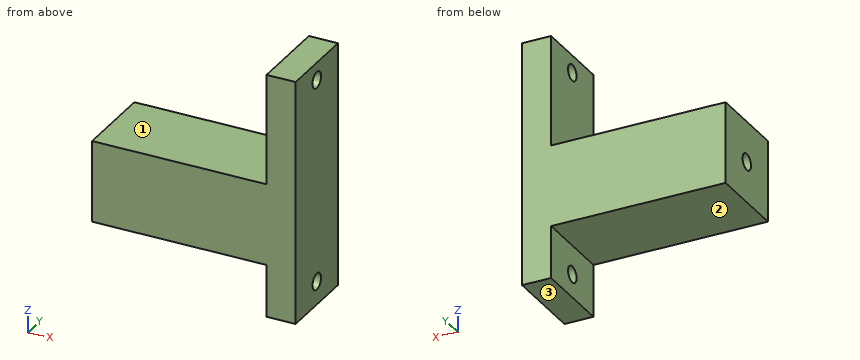
Autodesk Inventor part; units mm, degrees
ref_plane "YZ Plane" through (0, 0, 0) normal (1, 0, 0) x (0, 1, 0)
ref_plane "XZ Plane" through (0, 0, 0) normal (0, 1, 0) x (-1, 0, 0)
ref_plane "XY Plane" through (0, 0, 0) normal (0, 0, 1) x (1, 0, 0)
sketch "Sketch1" plane through (0, 0, 0) normal (1, 0, 0) x (0, 1, 0)
  line L0 (0, 0) -> (14, 0)
  line L1 (14, 0) -> (14, -42)
  line L2 (14, -42) -> (0, -42)
  line L3 (0, -42) -> (0, 0)
  line L4 (14, -19) -> (0, -19)
  line L5 (0, -19) -> (0, -33)
  line L6 (0, -33) -> (14, -33)
  line L7 (14, -33) -> (14, -19)
  circle A0 centre (7, -3) radius 1.4
  circle A1 centre (7, -38) radius 1.4
  point P0 (14, -33)
  point P1 (0, -19)
  dimension "d10" = 14
  dimension "d11" = 42
  dimension "d12" = 14
  dimension "d14" = 2.8
  dimension "d15" = 2.8
  dimension "d16" = 35
  dimension "d17" = 4
  dimension "d18" = 5
extrude "Extrusion1" add sketch "Sketch1" along normal blind 5 contours L0 L1 L4 L3 | L4 L1 L6 L3 | L6 L1 L2 L3 | A0 | A1
extrude "Extrusion2" add sketch "Sketch1" against normal blind 30 contours L4 L1 L6 L3
sketch "Sketch4" plane through (-30, 0, 0) normal (-1, 0, 0) x (0, 0, 1)
  line L0 (0, 0) -> (-42, 0)
  line L1 (-19, 14) -> (-19, 0)
  circle A0 centre (-26, 7) radius 1.4
  dimension "d19" = 2.8
extrude "Extrusion5" cut sketch "Sketch4" against normal blind 10
extrude "Extrusion6" cut sketch "Sketch1" along normal blind 10 contours A0 | A1
properties part number "_3DPrint"
Part model, mm, in its own coordinate system. Face numbers are marked on the shaded views. A direction names the side the tool comes from. Round coordinates to 2 decimals unless told otherwise and drop trailing zeros. Loops run counter-clockwise (first coordinate to the right, second up) from the corner with the lowest first, then second, coordinate; pieces in that order, holes last.
Item 1: Drop flat-ended pins along their axis: P1, Ø1.5, axis at x = -1, y = 4, coming from the -Z side; P2, Ø4.5, axis at y = 7, z = -38, coming from the -X side. Give the stop position or say it passes through.
Item 2: Cut at B-B, the plane y = 7. Give the cut face in (x, z).
Item 3: Cut at C-C, the plane x = 1. Give the cut face in (y, z), then the cut area to 3 significant figures.
Item 4: Cut at D-D, the plane y = 12. Give the cut face in (x, z), then the cut area to 3 significant figures.
Item 5: 3-axis set-ups, long thin cutter, end or side, ignore diameter. For the marked faces 1, 2 and 3: which of +Z, -Z, +X, -X, +Y, -Y reach the whole face in a straight line?
Item 6: Cut at A-A, the plane z = -3. Give the cut face in (x, y).
Item 7: Drill centre lines: line 1 (Z direction, x = 1.2, y = 7); line 2 (Y direction, x = 1, z = -3); line 3 (X direction, y = 1.75, z = -17). Where is each one in solid material? Low to high.
A:
1. P1: stops at z = -33
1. P2: stops at x = 0
2. outline: (-30, -33) - (0, -33) - (0, -36.6) - (5, -36.6) - (5, -4.4) - (0, -4.4) - (0, -19) - (-30, -19) - (-30, -24.6) - (-20, -24.6) - (-20, -27.4) - (-30, -27.4) - close; (0, -42) - (5, -42) - (5, -39.4) - (0, -39.4) - close; (0, -1.6) - (5, -1.6) - (5, 0) - (0, 0) - close
3. outline: (0, -42) - (14, -42) - (14, 0) - (0, 0) - close; hole circle Ø2.8 at (7, -38); hole circle Ø2.8 at (7, -3)
3. area: 576 mm2
4. outline: (-30, -33) - (0, -33) - (0, -42) - (5, -42) - (5, 0) - (0, 0) - (0, -19) - (-30, -19) - close
4. area: 630 mm2
5. face 1: +Z, -X, +Y, -Y
5. face 2: -Z, -X, +Y, -Y
5. face 3: -Z, +X, -X, +Y, -Y
6. outline: (0, 0) - (5, 0) - (5, 5.6) - (0, 5.6) - close; (0, 8.4) - (5, 8.4) - (5, 14) - (0, 14) - close
7. line 1: z = -42 to -39.4, -36.6 to -4.4, -1.6 to 0
7. line 2: y = 0 to 5.6, 8.4 to 14
7. line 3: x = 0 to 5
